Verification items for the finished model (mm, model axes). Face numbers are marked on the shaded views. Give positions to 0.01 mm unless a question says otherwise; leave off trailing zeros. Write each loop counter-clockwise with the first axis right and the second up, starting at its lowest first coordinate (ties: lowest second). Pieces come first, ordered by that corner, then holes.
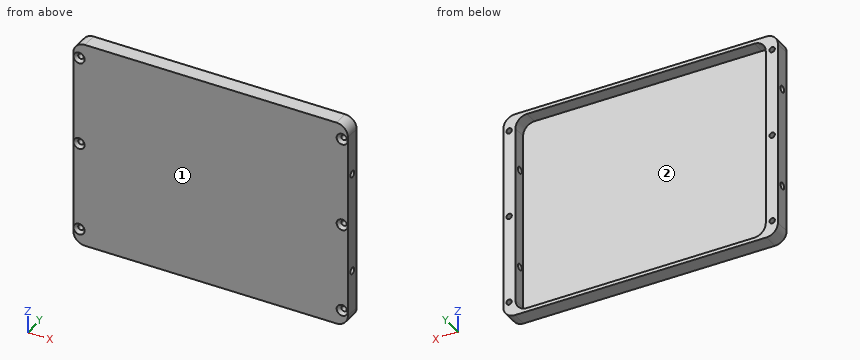
from build123d import *

# Parameters (mm, degrees)
SKETCH1_W                                         = 226.949
SKETCH1_H                                         = 171.45
BOSS_EXTRUDE1_DEPTH                               = 12.7
CUT_EXTRUDE1_DEPTH                                = 11.1125
F_1_4_28_TAPPED_HOLE1_REACH                       = 286.714
F_1_4_28_TAPPED_HOLE1_BORE_R                      = 2.7051
CSK_FOR_8_FLAT_HEAD_SOCKET_CAP_SCREW1_D           = 4.4958
CSK_FOR_8_FLAT_HEAD_SOCKET_CAP_SCREW1_CSINK_D     = 9.1186
CSK_FOR_8_FLAT_HEAD_SOCKET_CAP_SCREW1_CSINK_ANGLE = 82
FILLET1_R                                         = 9.525


with BuildPart() as part:
    # Sketch1 → Boss-Extrude1 (new body)
    with BuildSketch(Plane(origin=(0, 0, 0), x_dir=(1, 0, 0), z_dir=(0, 1, 0))):
        with Locations((113.4745, 85.725)):
            Rectangle(SKETCH1_W, SKETCH1_H)
    extrude(amount=BOSS_EXTRUDE1_DEPTH)

    # Sketch2 → Cut-Extrude1 (cut)
    with BuildSketch(Plane(origin=(0, 12.7, 0), x_dir=(1, 0, 0), z_dir=(0, 1, 0))):
        with BuildLine():
            Line((19.558, 2.921), (207.391, 2.921))
            ThreePointArc((207.391, 2.921), (214.126192091, 5.710807909), (216.916, 12.446))
            Line((216.916, 12.446), (216.916, 159.004))
            ThreePointArc((216.916, 159.004), (214.126192091, 165.739192091), (207.391, 168.529))
            Line((207.391, 168.529), (19.558, 168.529))
            ThreePointArc((19.558, 168.529), (12.822807909, 165.739192091), (10.033, 159.004))
            Line((10.033, 159.004), (10.033, 12.446))
            ThreePointArc((10.033, 12.446), (12.822807909, 5.710807909), (19.558, 2.921))
        make_face()
    extrude(amount=-CUT_EXTRUDE1_DEPTH, mode=Mode.SUBTRACT)

    # 1_4-28 Tapped Hole1 bore → 1_4-28 Tapped Hole1 (cut, up to next)
    with BuildSketch(Plane.ZY, mode=Mode.PRIVATE) as f_1_4_28_tapped_hole1_sk1:
        with Locations((-127, 6.35)):
            Circle(F_1_4_28_TAPPED_HOLE1_BORE_R)
    f_1_4_28_tapped_hole1_tool1 = extrude(f_1_4_28_tapped_hole1_sk1.sketch, amount=-F_1_4_28_TAPPED_HOLE1_REACH, mode=Mode.PRIVATE) & part.part
    # 1_4-28 Tapped Hole1 bore → 1_4-28 Tapped Hole1 (cut, up to next)
    with BuildSketch(Plane.ZY, mode=Mode.PRIVATE) as f_1_4_28_tapped_hole1_sk2:
        with Locations((-44.45, 6.35)):
            Circle(F_1_4_28_TAPPED_HOLE1_BORE_R)
    f_1_4_28_tapped_hole1_tool2 = extrude(f_1_4_28_tapped_hole1_sk2.sketch, amount=-F_1_4_28_TAPPED_HOLE1_REACH, mode=Mode.PRIVATE) & part.part
    f_1_4_28_tapped_hole1_1 = f_1_4_28_tapped_hole1_tool1.solids().sort_by_distance((0, 6.35, -127))[0]
    add(f_1_4_28_tapped_hole1_1, mode=Mode.SUBTRACT)
    f_1_4_28_tapped_hole1_2 = f_1_4_28_tapped_hole1_tool2.solids().sort_by_distance((0, 6.35, -44.45))[0]
    add(f_1_4_28_tapped_hole1_2, mode=Mode.SUBTRACT)
    f_1_4_28_tapped_hole1 = f_1_4_28_tapped_hole1_1 + f_1_4_28_tapped_hole1_2  # 1_4-28 Tapped Hole1 as one shape, for the pattern or mirror that repeats it

    # CSK for _8 Flat Head Socket Cap Screw1 (through all)
    with Locations(Plane.XZ):
        with Locations((4.7625, -12.7), (4.7625, -85.725), (4.7625, -158.75)):
            csk_for_8_flat_head_socket_cap_screw1 = CounterSinkHole(CSK_FOR_8_FLAT_HEAD_SOCKET_CAP_SCREW1_D / 2, CSK_FOR_8_FLAT_HEAD_SOCKET_CAP_SCREW1_CSINK_D / 2, counter_sink_angle=CSK_FOR_8_FLAT_HEAD_SOCKET_CAP_SCREW1_CSINK_ANGLE)

    # Mirror1: 1_4-28 Tapped Hole1, CSK for _8 Flat Head Socket Cap Screw1 across plane
    add(f_1_4_28_tapped_hole1.mirror(Plane(origin=(113.4745, 0, 0), x_dir=(0, 0, 1), z_dir=(1, 0, 0))), mode=Mode.SUBTRACT)
    add(csk_for_8_flat_head_socket_cap_screw1.mirror(Plane(origin=(113.4745, 0, 0), x_dir=(0, 0, 1), z_dir=(1, 0, 0))), mode=Mode.SUBTRACT)

    # Fillet1
    fillet1_edges = [part.edges().sort_by_distance(p)[0] for p in [
        (0, 6.35, -171.45),
        (226.949, 6.35, -171.45),
        (226.949, 6.35, 0),
        (0, 6.35, 0),
    ]]
    fillet(fillet1_edges, radius=FILLET1_R)


solid = part.part
Item 1: Sectioned sample at B-B on x = 36. Record the cut outline in (y, z), then the cut area to 3 significant figures.
Answer key:
outline: (0, -171.45) - (12.7, -171.45) - (12.7, -168.53) - (1.59, -168.53) - (1.59, -2.92) - (12.7, -2.92) - (12.7, 0) - (0, 0) - close
area: 337 mm2
Item 2: Scan lines: line 1 along X through (y, z) = (5.25, -12.7); line 2 along X through (y, z) = (7.5, -107); line 3 along Z through (x, y) = (108, 10). Record each from-to range of solid material in increasing order.
Answer key:
line 1: x = 0 to 2.51, 7.01 to 10.03, 216.92 to 219.94, 224.43 to 226.95
line 2: x = 0 to 10.03, 216.92 to 226.95
line 3: z = -171.45 to -168.53, -2.92 to 0
Item 3: Release check for a two-part mould opening along X. For the marked faces 1 and 2 record: released by +X, released by -X, zero draft, split by the parting line, or undercut.
Answer key:
face 1: zero draft
face 2: undercut
Item 4: Sectioned sample at D-D on z = -97. Record the cut outline in (x, y).
Answer key:
outline: (0, 0) - (226.95, 0) - (226.95, 12.7) - (216.92, 12.7) - (216.92, 1.59) - (10.03, 1.59) - (10.03, 12.7) - (0, 12.7) - close
Item 5: Sectioned sample at A-A on z = -44.45. Record the cut outline in (x, y).
Answer key:
outline: (0, 0) - (226.95, 0) - (226.95, 3.64) - (216.92, 3.64) - (216.92, 1.59) - (10.03, 1.59) - (10.03, 3.64) - (0, 3.64) - close; (0, 9.06) - (10.03, 9.06) - (10.03, 12.7) - (0, 12.7) - close; (216.92, 9.06) - (226.95, 9.06) - (226.95, 12.7) - (216.92, 12.7) - close
Item 6: Sectioned sample at C-C on y = 6.35. State how many separate pieces and enclosed holes the cut face has, then the cut area to 3 significant figures.
Answer key:
separate pieces: 4
enclosed holes: 6
area: 4,340 mm2
Item 7: Depth check by flat-ended pin: pin 1 (4 mm diameter, centred on x = 203, z = -60.5, fed in from +Y); pin 2 (2 mm diameter, centred on x = 146.5, z = -31, fed in from -Y); pin 3 (6 mm diameter, centred on x = 4.76, z = -85.72, fed in from -Y). Enter the tip coordinate at first touch or a pass-through.
Answer key:
pin 1: stops at y = 1.59
pin 2: stops at y = 0
pin 3: stops at y = 1.79
